Verification items for the finished model (mm, model axes). Face numbers are marked on the shaded views. A direction names the side the tool comes from. Give positions to 0.01 mm unless a question says otherwise; leave off trailing zeros. Loops run counter-clockwise (first coordinate to the right, second up) from the corner with the lowest first, then second, coordinate; pieces in that order, holes last. Notation, with made-up numbers: M 67.25,28 L 126.25,28 A26 cw 126.25,42 Z; hole C -4,46 d5. An arc over 180 degrees is marked long. Answer in a Markdown table with one row per item.
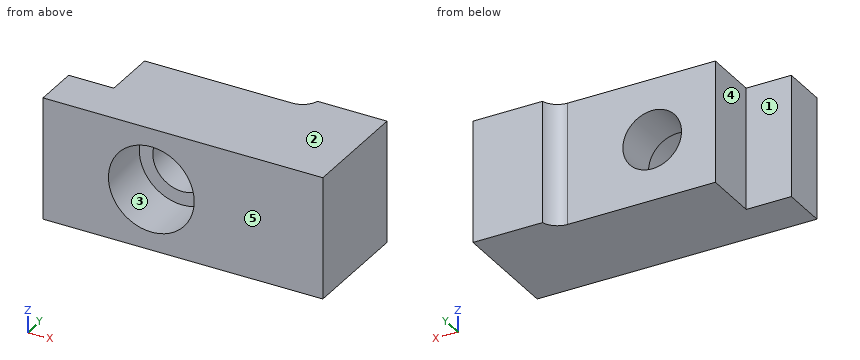
```python
from build123d import *

# Parameters (mm, degrees)
SKETCH2_W             = 62
SKETCH2_H             = 27
BOSS_EXTRUDE1_DEPTH   = 25
CUT_EXTRUDE1_DEPTH    = 28
SKETCH4_R             = 6.5
CUT_EXTRUDE2_DEPTH    = 26
BODY_MOVE_COPY1_ANGLE = 180
BOSS_EXTRUDE2_DEPTH   = 27
SKETCH6_R             = 9.5
CUT_EXTRUDE3_DEPTH    = 12


with BuildPart() as part:
    # Sketch2 → Boss-Extrude1 (new body)
    with BuildSketch(Plane(origin=(0, 0, 0), x_dir=(1, 0, 0), z_dir=(0, 1, 0))):
        Rectangle(SKETCH2_W, SKETCH2_H)
    extrude(amount=BOSS_EXTRUDE1_DEPTH)

    # Sketch3 → Cut-Extrude1 (cut, through all)
    with BuildSketch(Plane.XY.offset(13.5)):
        Polygon((-31, 0), (23.611888282, 0), (23.611888282, 3), (-21, 3), (-21, 15), (-31, 15), align=None)
    extrude(amount=-CUT_EXTRUDE1_DEPTH, mode=Mode.SUBTRACT)

    # Sketch4 → Cut-Extrude2 (cut, through all)
    with BuildSketch(Plane(origin=(0, 25, 0), x_dir=(1, 0, 0), z_dir=(0, 1, 0))):
        with Locations((-7, 0)):
            Circle(SKETCH4_R)
    extrude(amount=-CUT_EXTRUDE2_DEPTH, mode=Mode.SUBTRACT)


with BuildPart() as part_1:
    # Body-Move/Copy1: moved
    add(part.part.rotate(Axis((0, 12.5, 0), (1, 0, 0)), BODY_MOVE_COPY1_ANGLE))

    # Sketch5 → Boss-Extrude2 (add)
    with BuildSketch(Plane.XY.offset(13.5)):
        with BuildLine():
            Line((23.611888282, 25), (15.6, 25))
            ThreePointArc((15.6, 25), (14.176506397, 22.83772234), (11.727016654, 22))
            Line((11.727016654, 22), (23.611888282, 22))
            Line((23.611888282, 22), (23.611888282, 25))
        make_face()
    extrude(amount=-BOSS_EXTRUDE2_DEPTH)

    # Sketch6 → Cut-Extrude3 (cut)
    with BuildSketch(Plane.XZ):
        with Locations((-7, 0)):
            Circle(SKETCH6_R)
    extrude(amount=-CUT_EXTRUDE3_DEPTH, mode=Mode.SUBTRACT)


solid = part_1.part
```
Item 1: Sectioned sample at B-B (x = -7). Record the cut outline in (y, z), and give its area (3 significant figures).
Reported:
| item | result |
|---|---|
| outline | M 0,-13.5 L 22,-13.5 L 22,-6.5 L 12,-6.5 L 12,-9.5 L 0,-9.5 Z; M 0,9.5 L 12,9.5 L 12,6.5 L 22,6.5 L 22,13.5 L 0,13.5 Z |
| area | 236 mm^2 |
Item 2: Go/stop test with flat-tipped pins: pin 1 (5 mm diameter, centred on x = -2, z = -2.5, fed in from -Y); pin 2 (4 mm diameter, centred on y = 16.5, z = 10, fed in from -X); pin 3 (13.5 mm diameter, centred on x = -6, z = -1.5, fed in from +Y). Record where each tip stops, or that it passes through.
Reported:
| item | result |
|---|---|
| pin 1 | stops at y = 12 |
| pin 2 | stops at x = -21 |
| pin 3 | stops at y = 22 |
Item 3: Release check for a two-part mould opening along Z. For the marked faces 1, 2 and 3 record: released by +Z, released by -Z, zero draft, split by the parting line, or undercut.
Reported:
| item | result |
|---|---|
| face 1 | zero draft |
| face 2 | released by +Z |
| face 3 | undercut |
Item 4: Scan lines: L1, parallel to Z at x = -7, y = 7.5; L2, parallel to Z at x = -7, y = 16.5; L3, parallel to X at y = 8, z = -0.5. Record each from-to range of solid material in increasing order. Write a range as [from, to].
Reported:
| item | result |
|---|---|
| L1 | z = [-13.5, -9.5], [9.5, 13.5] |
| L2 | z = [-13.5, -6.5], [6.5, 13.5] |
| L3 | x = [-31, -16.49], [2.49, 31] |
Item 5: Tool access check on the marked faces 4 and 5. Record the directions out of +Z, -Z, +X, -X, +Y, -Y that give a thin tool (end or side, any length) a straight path to the whole face; none if there is none.
Reported:
| item | result |
|---|---|
| face 4 | +Z, -Z, -X, +Y |
| face 5 | +Z, -Z, +X, -X, -Y |
Item 6: Sectioned sample at D-D (z = -7.75). Record the cut outline in (x, y).
Reported:
| item | result |
|---|---|
| outline | M -31,0 L -12.49,0 L -12.49,12 L -1.51,12 L -1.51,0 L 31,0 L 31,25 L 15.6,25 A4 cw 11.73,22 L -21,22 L -21,10 L -31,10 Z |
Item 7: Sectioned sample at A-A (z = 0). Record the cut outline in (x, y).
Reported:
| item | result |
|---|---|
| outline | M -31,0 L -16.5,0 L -16.5,12 L -13.5,12 L -13.5,22 L -21,22 L -21,10 L -31,10 Z; M -0.5,12 L 2.5,12 L 2.5,0 L 31,0 L 31,25 L 15.6,25 A4 cw 11.73,22 L -0.5,22 Z |
Item 8: Sectioned sample at C-C (y = 3.5). Record the cut outline in (x, z).
Reported:
| item | result |
|---|---|
| outline | M -31,-13.5 L 31,-13.5 L 31,13.5 L -31,13.5 Z; hole C -7,0 d19 |
